Could you check a few things on this model? Use its own coordinates, in mm. A direction names the side the tool comes from. Round coordinates to 2 decimals unless told otherwise and drop trailing zeros. Loops run counter-clockwise (first coordinate to the right, second up) from the corner with the lowest first, then second, coordinate; pieces in that order, holes last.
from build123d import *

# Parameters (mm, degrees)
SKETCH1_W                  = 20
SKETCH1_H                  = 20
SKETCH1_W_2                = 8
BOSS_EXTRUDE1_DEPTH        = 10
F_4_0_209_DIAMETER_HOLE1_D = 5.3086
SKETCH1_3_W                = 8
SKETCH1_3_H                = 20
BOSS_EXTRUDE2_DEPTH        = 10


with BuildPart() as part:
    # Sketch1 → Boss-Extrude1 (new body)
    with BuildSketch(Plane.XY):
        Rectangle(SKETCH1_W, SKETCH1_H)
        with Locations((0, 20)):
            Rectangle(SKETCH1_W_2, SKETCH1_H)
    extrude(amount=BOSS_EXTRUDE1_DEPTH)

    # 4 _0.209_ Diameter Hole1 (through all)
    with Locations(Plane.XY.offset(10)):
        with Locations((0, 0)):
            Hole(F_4_0_209_DIAMETER_HOLE1_D / 2)

    # Sketch1_3 → Boss-Extrude2 (add)
    with BuildSketch(Plane.XY):
        with Locations((0, 20)):
            Rectangle(SKETCH1_3_W, SKETCH1_3_H)
    extrude(amount=-BOSS_EXTRUDE2_DEPTH)


solid = part.part
Item 1: If we section it at D-D, the plane z = -2.75: Please give me the cut outline in (x, y).
Results list:
outline: (-4, 10) - (4, 10) - (4, 30) - (-4, 30) - close
Item 2: For faces 5 (the flat face through (10, 0, 5)), 6 (the flat face through (-7, 10, 5)), 7 (the flat face through (4, 20, 0)), 8 (the flat face through (-2, -2, 0)), which set-ups out of +Z, -Z, +X, -X, +Y, -Y let a thin tool reach every point of the face, with its end or its side?
Results list:
face 5: +Z, -Z, +X, +Y, -Y
face 6: +Z, -Z, -X, +Y
face 7: +Z, -Z, +X, +Y
face 8: -Z, +X, -X, -Y
Item 3: If we section it at B-B, the plane x = 0: Please give me the cut outline in (y, z).
Results list:
outline: (-10, 0) - (-2.65, 0) - (-2.65, 10) - (-10, 10) - close; (2.65, 0) - (10, 0) - (10, -10) - (30, -10) - (30, 10) - (2.65, 10) - close
Item 4: Will these pins go through, and if not, where does the flat tip stop? pin 1 (4 mm diameter, centred on y = 17, z = -5, fed in from +X); pin 2 (10 mm diameter, centred on x = -1.5, y = 2.5, fed in from -Z); pin 3 (2 mm diameter, centred on x = 7, z = -2, fed in from +Y); pin 4 (9 mm diameter, centred on x = 0.5, z = -6.5, fed in from -Y).
Results list:
pin 1: stops at x = 4
pin 2: stops at z = 0
pin 3: passes through
pin 4: stops at y = 10
Item 5: If we section it at C-C, the plane y = 0: Please give me the cut outline in (x, z), then the cut area to 3 significant figures.
Results list:
outline: (-10, 0) - (-2.65, 0) - (-2.65, 10) - (-10, 10) - close; (2.65, 0) - (10, 0) - (10, 10) - (2.65, 10) - close
area: 147 mm2
Item 6: If we section it at A-A, the plane z = 4.25: Please give me the cut outline in (x, y).
Results list:
outline: (-10, -10) - (10, -10) - (10, 10) - (4, 10) - (4, 30) - (-4, 30) - (-4, 10) - (-10, 10) - close; hole circle Ø5.31 at (0, 0)
Item 7: We'd pull the mould along Y, two halves only. Please class faces 1 (the flat face through (7, 10, 5)), 2 (the flat face through (-10, 0, 5)), 3 (the flat face through (0, 10, -5)), 4 (the cylindrical face through (-2.53, 0.8, 4.93)): released by +Y, released by -Y, zero draft, split by the parting line, or undercut.
Results list:
face 1: released by +Y
face 2: zero draft
face 3: released by -Y
face 4: undercut
Item 8: If I drill on line 1 along X through (y, z) = (25.5, -3.5); line 2 along Y through (x, z) = (0, 5.5); line 3 along Z through (x, y) = (2.5, 4.5), over which ranges is the centre line in solid material (lowest first)?
Results list:
line 1: x = -4 to 4
line 2: y = -10 to -2.65, 2.65 to 30
line 3: z = 0 to 10
